Verification items for the finished model (mm, model axes). Face numbers are marked on the shaded views. Coordinates: 2 decimals unless noted, no trailing zeros. Write each loop counter-clockwise with the first axis right and the second up, starting at its lowest first coordinate (ties: lowest second). Pieces come first, ordered by that corner, then holes. Notation, with made-up numbers: (63, 20.5) -> (82, 20.5) arc R18 ccw to (82, 39.5) -> close; hole circle Ø5 at (-15.5, 9). An arc over 180 degrees is marked (long way). Use a Markdown table: item, result. Add a question column.
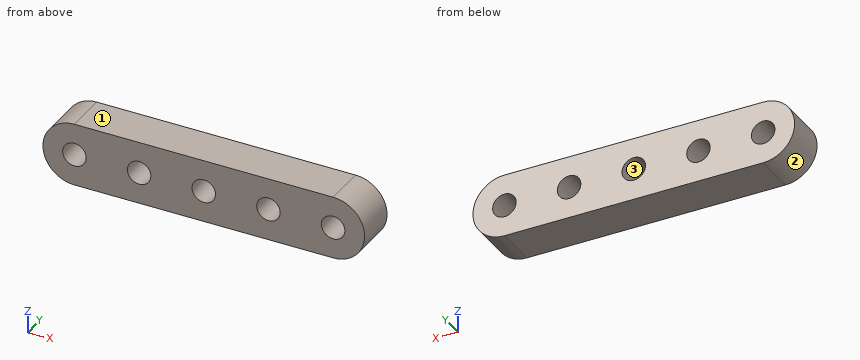
from build123d import *

# Parameters (mm, degrees)
SKETCH1_R           = 1.778
BOSS_EXTRUDE1_DEPTH = 6.35


with BuildPart() as part:
    # Sketch1 → Boss-Extrude1 (new body)
    with BuildSketch(Plane(origin=(0, 6.35, 0), x_dir=(1, 0, 0), z_dir=(0, 1, 0))):
        with BuildLine():
            Line((19.558, 4.7625), (-19.558, 4.7625))
            ThreePointArc((-19.558, 4.7625), (-24.3205, 0), (-19.558, -4.7625))
            Line((-19.558, -4.7625), (19.558, -4.7625))
            ThreePointArc((19.558, -4.7625), (24.3205, 0), (19.558, 4.7625))
        make_face()
        with Locations((19.558, 0)):
            Circle(SKETCH1_R, mode=Mode.SUBTRACT)
        with Locations((9.779, 0)):
            Circle(SKETCH1_R, mode=Mode.SUBTRACT)
        Circle(SKETCH1_R, mode=Mode.SUBTRACT)
        with Locations((-9.779, 0)):
            Circle(SKETCH1_R, mode=Mode.SUBTRACT)
        with Locations((-19.558, 0)):
            Circle(SKETCH1_R, mode=Mode.SUBTRACT)
    extrude(amount=-BOSS_EXTRUDE1_DEPTH)


solid = part.part
1) Thickness scan on L1, parallel to X at y = 5, z = 0; L2, parallel to X at y = 5.25, z = 1; L3, parallel to Z at x = -9, y = 1.25. Record the ranges inside material, lowest first.
2) Release check for a two-part mould opening along X. For the marked faces 1, 2 and 3 record: released by +X, released by -X, zero draft, split by the parting line, or undercut.
3) Cross-section at A-A on y = 1. Record the boundary of the cut face in (x, z) (1 decimal).
4) Gauge pin test, flat ends, axial feed: pin 1 (3 mm diameter, centred on y = 5, z = -2, fed in from +X); pin 2 (2 mm diameter, centred on x = -19.558, z = 0, fed in from -Y). Record the tip position at first contact, or that the pin passes through.
5) Cross-section at D-D on x = 8.5. Record the boundary of the cut face in (y, z).
6) Cross-section at C-C on x = 0. Record the boundary of the cut face in (y, z), then the cut area to 3 significant figures.
7) Cross-section at B-B on z = 0. Record the boundary of the cut face in (x, y).
Returned:
| question | item | result |
|---|---|---|
| 1 | L1 | x = -24.32 to -21.34, -17.78 to -11.56, -8 to -1.78, 1.78 to 8, 11.56 to 17.78, 21.34 to 24.32 |
| 1 | L2 | x = -24.21 to -21.03, -18.09 to -11.25, -8.31 to -1.47, 1.47 to 8.31, 11.25 to 18.09, 21.03 to 24.21 |
| 1 | L3 | z = -4.76 to -1.6, 1.6 to 4.76 |
| 2 | face 1 | zero draft |
| 2 | face 2 | released by -X |
| 2 | face 3 | undercut |
| 3 | outline | (-19.6, -4.8) -> (19.6, -4.8) arc R4.8 ccw to (19.6, 4.8) -> (-19.6, 4.8) arc R4.8 ccw to start; hole circle Ø3.6 at (-19.6, 0); hole circle Ø3.6 at (-9.8, 0); hole circle Ø3.6 at (0, 0); hole circle Ø3.6 at (9.8, 0); hole circle Ø3.6 at (19.6, 0) |
| 4 | pin 1 | stops at x = 24.29 |
| 4 | pin 2 | passes through |
| 5 | outline | (0, -4.76) -> (6.35, -4.76) -> (6.35, -1.24) -> (0, -1.24) -> close; (0, 1.24) -> (6.35, 1.24) -> (6.35, 4.76) -> (0, 4.76) -> close |
| 6 | outline | (0, -4.76) -> (6.35, -4.76) -> (6.35, -1.78) -> (0, -1.78) -> close; (0, 1.78) -> (6.35, 1.78) -> (6.35, 4.76) -> (0, 4.76) -> close |
| 6 | area | 37.9 mm² |
| 7 | outline | (-24.32, 0) -> (-21.34, 0) -> (-21.34, 6.35) -> (-24.32, 6.35) -> close; (-17.78, 0) -> (-11.56, 0) -> (-11.56, 6.35) -> (-17.78, 6.35) -> close; (-8, 0) -> (-1.78, 0) -> (-1.78, 6.35) -> (-8, 6.35) -> close; (1.78, 0) -> (8, 0) -> (8, 6.35) -> (1.78, 6.35) -> close; (11.56, 0) -> (17.78, 0) -> (17.78, 6.35) -> (11.56, 6.35) -> close; (21.34, 0) -> (24.32, 0) -> (24.32, 6.35) -> (21.34, 6.35) -> close |
